```python
from build123d import *

# Parameters (mm, degrees)
SKETCH_1_W          = 150.689919998
SKETCH_1_H          = 63.936654908
EXTRUDE_1_DEPTH     = 6
FILLET_6_R          = 5
FILLET_7_R          = 5
FILLET_8_R          = 5
FILLET_9_R          = 5
SKETCH_2_W          = 7.93449938
SKETCH_2_H          = 1.809622666
CUT_EXTRUDE_1_DEPTH = 11
SKETCH_3_W          = 6.791001318
SKETCH_3_H          = 0.456984439
EXTRUDE_4_DEPTH     = 10
SKETCH_4_R          = 1
CUT_EXTRUDE_2_DEPTH = 10
SKETCH_7_R          = 0.626407846
EXTRUDE_5_DEPTH     = 5.887149494
SKETCH_11_R         = 0.5
CUT_EXTRUDE_4_DEPTH = 10
SKETCH_12_R         = 23.442239877
EXTRUDE_6_DEPTH     = 3
FILLET_11_R         = 5
EXTRUDE_7_DEPTH     = 2
SKETCH_16_R         = 0.5
CUT_EXTRUDE_5_DEPTH = 7


with BuildPart() as part:
    # 草图1 → 凸台-拉伸1 (new body)
    with BuildSketch(Plane(origin=(0, 0, 0), x_dir=(1, 0, 0), z_dir=(0, 1, 0))):
        with Locations((14.918552812, -2.00585584)):
            Rectangle(SKETCH_1_W, SKETCH_1_H)
    extrude(amount=EXTRUDE_1_DEPTH)

    # 圆角6
    fillet_6_edges = [part.edges().sort_by_distance(p)[0] for p in [
        (90.263512811, 3, -29.962471614),
    ]]
    fillet(fillet_6_edges, radius=FILLET_6_R)

    # 圆角7
    fillet_7_edges = [part.edges().sort_by_distance(p)[0] for p in [
        (90.263512811, 3, 33.974183294),
    ]]
    fillet(fillet_7_edges, radius=FILLET_7_R)

    # 圆角8
    fillet_8_edges = [part.edges().sort_by_distance(p)[0] for p in [
        (-60.426407187, 3, 33.974183294),
    ]]
    fillet(fillet_8_edges, radius=FILLET_8_R)

    # 圆角9
    fillet_9_edges = [part.edges().sort_by_distance(p)[0] for p in [
        (-60.426407187, 3, -29.962471614),
    ]]
    fillet(fillet_9_edges, radius=FILLET_9_R)

    # 草图2 → 切除-拉伸1 (cut)
    with BuildSketch(Plane.ZY.offset(60.426407187)):
        with Locations((1.518649738, 3.03572559)):
            Rectangle(SKETCH_2_W, SKETCH_2_H)
    extrude(amount=-CUT_EXTRUDE_1_DEPTH, mode=Mode.SUBTRACT)

    # 草图3 → 凸台-拉伸4 (add)
    with BuildSketch(Plane.ZY.offset(49.426407187)):
        with Locations((1.631220099, 3.18901263)):
            Rectangle(SKETCH_3_W, SKETCH_3_H)
    extrude(amount=EXTRUDE_4_DEPTH)

    # 草图4 → 切除-拉伸2 (cut)
    with BuildSketch(Plane.ZY.offset(60.426407187)):
        with Locations((13.072394448, 3.110545162)):
            Circle(SKETCH_4_R)
        with Locations((16.065231934, 3.110545162)):
            Circle(SKETCH_4_R)
        with Locations((19.406073778, 3.110545162)):
            Circle(SKETCH_4_R)
        with Locations((22.468512134, 3.110545162)):
            Circle(SKETCH_4_R)
        with Locations((10.079556963, 3.110545162)):
            Circle(SKETCH_4_R)
        with Locations((25.391748748, 3.110545162)):
            Circle(SKETCH_4_R)
    extrude(amount=-CUT_EXTRUDE_2_DEPTH, mode=Mode.SUBTRACT)

    # 草图7 → 凸台-拉伸5 (add)
    with BuildSketch(Plane.ZY.offset(50.426407187)):
        with BuildLine():
            Line((-21.86724317, 4.160702093), (-5.58063918, 4.160702093))
            ThreePointArc((-5.58063918, 4.160702093), (-4.53048225, 3.110545162), (-5.58063918, 2.060388231))
            Line((-5.58063918, 2.060388231), (-21.86724317, 2.060388231))
            ThreePointArc((-21.86724317, 2.060388231), (-22.9174001, 3.110545162), (-21.86724317, 4.160702093))
        make_face()
        with Locations((-21.86724317, 3.110545162)):
            Circle(SKETCH_7_R, mode=Mode.SUBTRACT)
    extrude(amount=EXTRUDE_5_DEPTH)

    # 草图11 → 切除-拉伸4 (cut)
    with BuildSketch(Plane.ZY.offset(60.426407187)):
        with Locations((-22.772054502, 3.417504849)):
            Circle(SKETCH_11_R)
    extrude(amount=-CUT_EXTRUDE_4_DEPTH, mode=Mode.SUBTRACT)

    # 草图12 → 凸台-拉伸6 (add)
    with BuildSketch(Plane.XZ):
        with Locations(Location((58.895102962, 2.00585584, 0), (0, 0, 90))):
            Circle(SKETCH_12_R)
    extrude(amount=EXTRUDE_6_DEPTH)

    # 圆角11
    # the kernel refuses this fillet: 5 mm, written as the material it takes off along each edge
    with BuildSketch(Plane(origin=(58.895102962, -3, 2.00585584), x_dir=(0, 0, 1), z_dir=(1, 0, 0))) as fillet_11_piece_1:
        with BuildLine():
            CenterArc((18.859664182, -5), FILLET_11_R, 23.578178478, 66.421821522)
            Line((18.859664182, 0), (18.859664182, 0.1))
            Line((18.859664182, 0.1), (23.442239877, 0.1))
            Line((23.442239877, 0.1), (23.542239877, 0))
            ThreePointArc((23.542239877, 0), (23.542239877, -1.5), (23.533891391, -2.96))
            Line((23.533891391, -2.96), (23.442239877, -3))
        make_face()
    revolve(axis=Axis((58.895102962, -3, 2.00585584), (0, -1, 0)), mode=Mode.SUBTRACT)

    # 草图15 → 凸台-拉伸7 (add)
    with BuildSketch(Plane.XY.offset(33.974183294)):
        with BuildLine():
            Line((72.53746341, 1.907291866), (56.006132514, 1.907291866))
            ThreePointArc((56.006132514, 1.907291866), (54.91342438, 3), (56.006132514, 4.092708134))
            Line((56.006132514, 4.092708134), (72.53746341, 4.092708134))
            ThreePointArc((72.53746341, 4.092708134), (73.630171544, 3), (72.53746341, 1.907291866))
        make_face()
        with BuildLine():
            Line((45.092244156, 1.907291866), (33.05486729, 1.907291866))
            ThreePointArc((33.05486729, 1.907291866), (31.962159155, 3), (33.05486729, 4.092708134))
            Line((33.05486729, 4.092708134), (45.092244156, 4.092708134))
            ThreePointArc((45.092244156, 4.092708134), (46.18495229, 3), (45.092244156, 1.907291866))
        make_face()
    extrude(amount=EXTRUDE_7_DEPTH)

    # 草图16 → 切除-拉伸5 (cut)
    with BuildSketch(Plane(origin=(90.263512811, 0, 0), x_dir=(0, 0, -1), z_dir=(1, 0, 0))):
        with Locations((0, 3)):
            Circle(SKETCH_16_R)
        with Locations((1.488767231, 3)):
            Circle(SKETCH_16_R)
        with Locations((-2.00585584, 3)):
            Circle(SKETCH_16_R)
        with Locations((-3.848597666, 3)):
            Circle(SKETCH_16_R)
    extrude(amount=-CUT_EXTRUDE_5_DEPTH, mode=Mode.SUBTRACT)


solid = part.part
```
Model file for the job. Use its own axes, mm. A direction names the side the tool comes from. Give positions to 0.01 mm unless a question says otherwise; leave off trailing zeros.
1) Mould opens along Z. For faces 3 (the cylindrical face through (88.84, 3.04, 32.47)), 4 (the flat face through (-54, 3.418, 2)), 5 (the cylindrical face through (-59, 3.04, -28.46)), 6 (the flat face through (-3, 0, 2)) say: +Z half, -Z half, draft (parallel to the pull), parting line (faces both ways), or undercut.
2) Wall check: probe 1 along Y at (x, z) = (-40.5, -23); probe 2 along Z at (x, y) = (39.5, 1.75); probe 3 along X at (y, z) = (3.25, 10). Give the ranges that are in metal, low to high.
3) Pin check, flat tips, straight feed: pin 1 (1.6 mm diameter, centred on y = 3, z = 19.5, fed in from -X); pin 2 (0.5 mm diameter, centred on y = 3, z = 2, fed in from +X); pin 3 (2 mm diameter, centred on y = 3, z = 13.5, fed in from -X); pin 4 (1.5 mm diameter, centred on x = 27, z = 5, fed in from -Y). Stop position of each tip, or through.
4) 3-axis set-ups, long thin cutter, end or side, ignore diameter. For faces 1 (the flat face through (-54, 2.961, 2)), 2 (the flat face through (59, -3, 2)): which of +Z, -Z, +X, -X, +Y, -Y reach the whole face in a straight line?
Computed:
1. face 3: +Z half
1. face 4: undercut
1. face 5: -Z half
1. face 6: draft
2. probe 1: y = 0 to 6
2. probe 2: z = -29.96 to 33.97
2. probe 3: x = -50.43 to 90.26
3. pin 1: stops at x = -50.43
3. pin 2: stops at x = 83.26
3. pin 3: stops at x = -60.43
3. pin 4: stops at y = 0
4. face 1: -X
4. face 2: +Z, -Z, +X, -X, -Y
